from build123d import *

# Parameters (mm, degrees)
DODANIE_WYCI_GNI_CIE1_DEPTH = 220
DODANIE_WYCI_GNI_CIE2_DEPTH = 20
SZKIC3_W                    = 160
SZKIC3_H                    = 14
DODANIE_WYCI_GNI_CIE3_DEPTH = 20
WYTNIJ_WYCI_GNI_CIE1_DEPTH  = 781.773516846


with BuildPart() as part:
    # Szkic1 → Dodanie-wyciągnięcie1 (new body)
    with BuildSketch(Plane.XY):
        Polygon((600, 0), (747.721162952, 26.04722665), (747.721162952, 46.04722665), (600, 20), (0, 20), (0, 0), align=None)
    extrude(amount=DODANIE_WYCI_GNI_CIE1_DEPTH)

    # Szkic2 → Dodanie-wyciągnięcie2 (add)
    with BuildSketch(Plane(origin=(0, 20, 0), x_dir=(1, 0, 0), z_dir=(0, 1, 0))):
        Polygon((1, -1), (599, -1), (599, 0), (0, 0), (0, -220), (599, -220), (599, -219), (1, -219), align=None)
    extrude(amount=DODANIE_WYCI_GNI_CIE2_DEPTH)

    # Szkic3 → Dodanie-wyciągnięcie3 (add)
    with BuildSketch(Plane.XZ):
        with Locations((520, 213)):
            Rectangle(SZKIC3_W, SZKIC3_H)
        with Locations((520, 7)):
            Rectangle(SZKIC3_W, SZKIC3_H)
    extrude(amount=DODANIE_WYCI_GNI_CIE3_DEPTH)

    # Szkic4 → Wytnij-wyciągnięcie1 (cut, through all)
    with BuildSketch(Plane.XY.offset(220)):
        with BuildLine():
            Line((585, -13), (455, -13))
            ThreePointArc((455, -13), (452, -10), (455, -7))
            Line((455, -7), (585, -7))
            ThreePointArc((585, -7), (588, -10), (585, -13))
        make_face()
    extrude(amount=-WYTNIJ_WYCI_GNI_CIE1_DEPTH, mode=Mode.SUBTRACT)


solid = part.part
Model file for the job. Use its own axes, mm. A direction names the side the tool comes from. Coordinates: 2 decimals unless noted, no trailing zeros. Write each loop counter-clockwise with the first axis right and the second up, starting at its lowest first coordinate (ties: lowest second). Pieces come first, ordered by that corner, then holes. Notation, with made-up numbers: (36.25, -14.5) - (49.25, -14.5) arc R17 cw to (49.25, 4.5) - close; hole circle Ø11 at (-22, -25). An arc over 180 degrees is marked (long way). Write each question's results on one line, items separated by ' | '. Start each with the question number.
1) Probe line 1 along Z through (x, y) = (368, 24); line 2 along Y through (x, z) = (301, 100); line 3 along Y through (x, z) = (648, 24). List the from-to ranges inside material, lowest first. Write a range as from..to.
2) Mould opens along Y. For faces 1 (the face through (521, -13, 213)), 2 (the face through (519, -20, 213)), 3 (the face through (440, -10, 7)) say: pulls with the +Y half, pulls with the -Y half, needs draft (parallel to the pull), parting line crosses it, or undercut.
3) Cut at A-A (z = 115.5). Write the cut outline in (x, y).
4) 3-axis set-ups, long thin cutter, end or side, ignore diameter. For faces 4 (the face through (519, -5, 14)), 5 (the face through (519, -7, 7)), 6 (the face through (600, -10, 213)): which of +Z, -Z, +X, -X, +Y, -Y reach the whole face in a straight line?
5) Cut at B-B (x = 405). Write the cut outline in (y, z).
6) Flat gauge pins, fed straight in: P1, Ø7, axis at x = 496, z = 9, coming from the +Y side; P2, Ø4, axis at y = -6, z = 211, coming from the +X side. Where does each tip first touch, or does it go through?
Returned:
1) line 1: 0..1, 219..220 | line 2: 0..20 | line 3: 8.46..28.46
2) face 1: undercut | face 2: pulls with the -Y half | face 3: needs draft
3) outline: (0, 0) - (600, 0) - (747.72, 26.05) - (747.72, 46.05) - (600, 20) - (1, 20) - (1, 40) - (0, 40) - close
4) face 4: +X, -X, -Y | face 5: +Z, -Z | face 6: +Z, -Z, +X, -Y
5) outline: (0, 0) - (40, 0) - (40, 1) - (20, 1) - (20, 219) - (40, 219) - (40, 220) - (0, 220) - close
6) P1: y = 20 | P2: x = 600
